The listing builds one solid part. Answer for the finished solid, in the listing's coordinates (mm). Face numbers are marked on the shaded views. A direction names the side the tool comes from. Round coordinates to 2 decimals unless told otherwise and drop trailing zeros. Loops run counter-clockwise (first coordinate to the right, second up) from the corner with the lowest first, then second, coordinate; pieces in that order, holes last. Notation, with made-up numbers: M 35,79.5 L 69,79.5 A23 cw 69,110.5 Z; hole C -22.5,76 d8. An arc over 180 degrees is marked long. Put each result on its own line as item: value. Start each with the question number.
(1) Which of the six approach directions +Z, -Z, +X, -X, +Y, -Y give full straight-line access (tool end or side, diameter ignored) to the marked faces 1, 2 and 3?
(2) Section C-C, the plane y = -1 is taken. Determine the outline of the cut face in (x, z), then the cut area to 3 significant figures.
(3) Straight lines are drawn through the part: line 1 (Z direction, x = 3, y = 0); line 2 (Z direction, x = 16, y = -13.5); line 3 (Y direction, x = 16, z = -24.5). For each, find the intervals that lie inside material, in ascending order.
(4) Determine the mould class of the marked faces 4, 5 and 6 for opening direction X: released by +X, released by -X, zero draft, split by the parting line, or undercut.
(5) Section A-A, the plane y = 10 is taken. Determine the outline of the cut face in (x, z).
(6) A flat-ended cylindrical pin translates along its axis: P1, Ø9.5, axis at x = -2.5, y = 7.5, coming from the +Z side. Find the tip coordinate at first contact, or state that the pin passes through.
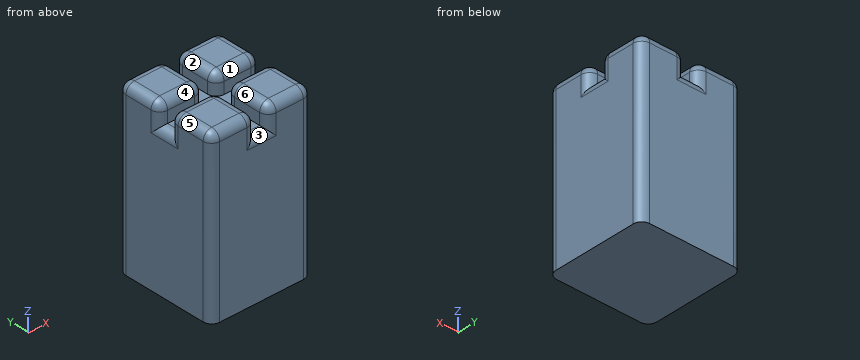
```python
from build123d import *

# Parameters (mm, degrees)
F0_W     = 38.1
F0_H     = 38.1
F2_DEPTH = 31.75
F4_W     = 4.572
F4_H     = 16.764
F3_W     = 16.764
F3_H     = 4.572
F3_W_2   = 4.572
F3_H_2   = 16.764
F5_DEPTH = 7.62
F6_R     = 3.2591265624


with BuildPart() as f2:
    # F0 (on Top) → F2 (new body, symmetric)
    with BuildSketch(Plane.XY):
        Rectangle(F0_W, F0_H)
    extrude(amount=F2_DEPTH, both=True)

    # F4 (on face) + F3 (on face) → F5 (cut)
    with BuildSketch(Plane.XY.offset(31.75)):
        with Locations((0, 10.668)):
            Rectangle(F4_W, F4_H)
    with BuildSketch(Plane.XY.offset(31.75)):
        with Locations((-10.668, 0)):
            Rectangle(F3_W, F3_H)
        Rectangle(F3_W_2, F3_H)
        with Locations((10.668, 0)):
            Rectangle(F3_W, F3_H)
        with Locations((0, -10.668)):
            Rectangle(F3_W_2, F3_H_2)
    extrude(amount=-F5_DEPTH, mode=Mode.SUBTRACT)

    # F6
    f6_edges = [f2.edges().sort_by_distance(p)[0] for p in [
        (10.668, 19.05, 31.75),
        (19.05, 10.668, 31.75),
        (19.05, 19.05, 0),
        (2.286, -10.668, 31.75),
        (10.668, 2.286, 31.75),
        (19.05, 0, 24.13),
        (19.05, 2.286, 27.94),
        (19.05, -2.286, 27.94),
        (19.05, -10.668, 31.75),
        (19.05, -19.05, 0),
        (10.668, -19.05, 31.75),
        (2.286, -19.05, 27.94),
        (0, -19.05, 24.13),
        (-2.286, -19.05, 27.94),
        (10.668, -2.286, 31.75),
        (-19.05, -10.668, 31.75),
        (-10.668, -2.286, 31.75),
        (-2.286, -10.668, 31.75),
        (-10.668, -19.05, 31.75),
        (-19.05, -2.286, 27.94),
        (-19.05, 0, 24.13),
        (-19.05, 2.286, 27.94),
        (-19.05, 10.668, 31.75),
        (-19.05, 19.05, 0),
        (-10.668, 19.05, 31.75),
        (-10.668, 2.286, 31.75),
        (-2.286, 19.05, 27.94),
        (2.286, 19.05, 27.94),
        (0, 19.05, 24.13),
        (-2.286, 2.286, 27.94),
        (-2.286, -2.286, 27.94),
        (2.286, 2.286, 27.94),
        (2.286, -2.286, 27.94),
        (-19.05, -19.05, 0),
        (-2.286, 10.668, 31.75),
        (2.286, 10.668, 31.75),
    ]]
    fillet(f6_edges, radius=F6_R)


solid = f2.part
```
Recorded:
1. face 1: +Z, +X, -X
1. face 2: +Z, +Y, -Y
1. face 3: +Z, -Y
2. outline: M -19.05,-31.75 L 19.05,-31.75 L 19.05,20.87 A3.26 ccw 15.79,24.13 L -15.79,24.13 A3.26 ccw -19.05,20.87 Z
2. area: 2,120 mm²
3. line 1: z = -31.75 to 24.13
3. line 2: z = -31.75 to 31.74
3. line 3: y = -19.04 to 19.04
4. face 4: zero draft
4. face 5: released by -X
4. face 6: undercut
5. outline: M -19.05,-31.75 L 19.05,-31.75 L 19.05,28.49 A3.26 ccw 15.79,31.75 L 5.55,31.75 A3.26 ccw 2.29,28.49 L 2.29,24.13 L -2.29,24.13 L -2.29,28.49 A3.26 ccw -5.55,31.75 L -15.79,31.75 A3.26 ccw -19.05,28.49 Z
6. P1: stops at z = 31.75
